Answer from the drawing. Dimensions are ordinates in mm from the lowest x, y and z of the part. A direction names the side the tool comes from. Round coordinates to 2 decimals unless told otherwise and drop trailing zeros. Order: outer loops, then holes, each group sorted by start corner. A loop starts at its lowest first (then second) coordinate and runs counter-clockwise, first axis right, second up.
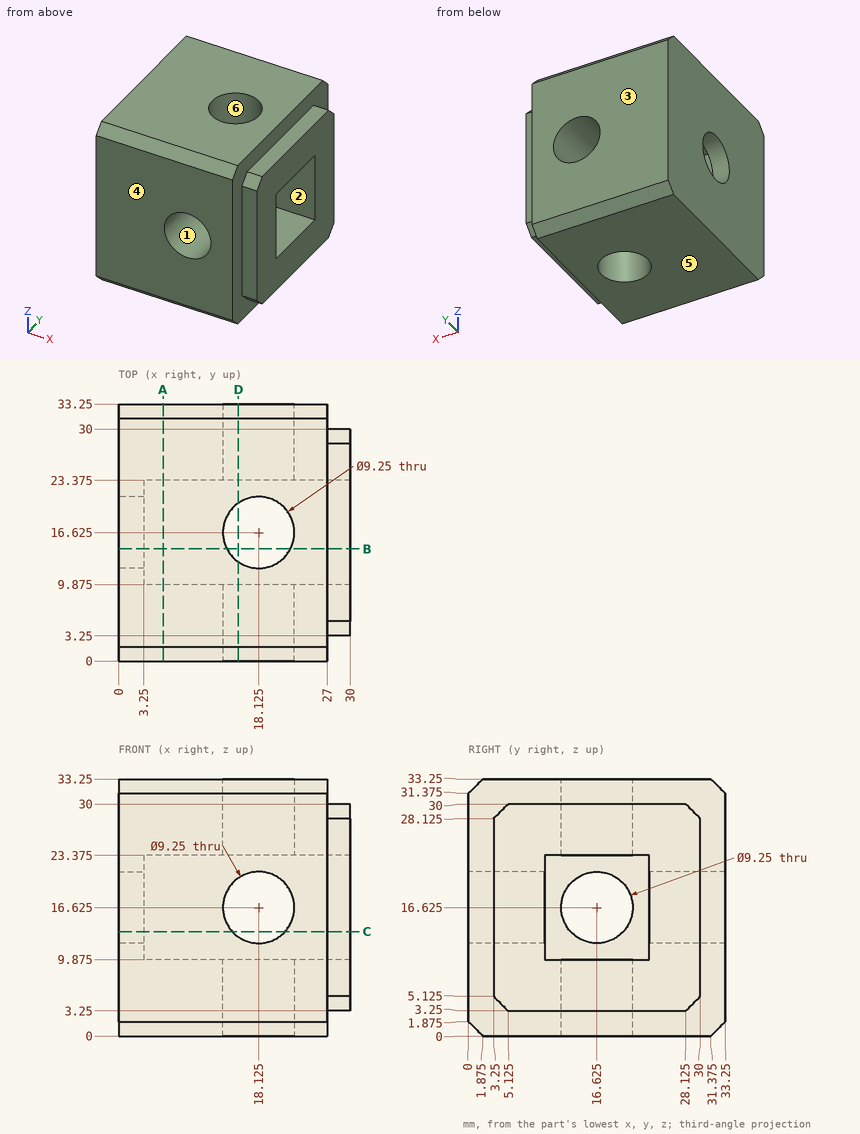
Q1. A cutting plane is placed at B-B, the plane y = 14.5. Give the vertices of the cut face in (x, z) (3 decimals).
Outcome:
outline: (0, 0) - (14.017, 0) - (14.017, 9.875) - (3.25, 9.875) - (3.25, 12.517) - (0, 12.517) - close; (0, 20.733) - (3.25, 20.733) - (3.25, 23.375) - (14.017, 23.375) - (14.017, 33.25) - (0, 33.25) - close; (22.233, 0) - (27, 0) - (27, 3.25) - (30, 3.25) - (30, 9.875) - (22.233, 9.875) - close; (22.233, 23.375) - (30, 23.375) - (30, 30) - (27, 30) - (27, 33.25) - (22.233, 33.25) - close
Q2. A cutting plane is placed at C-C, the plane z = 13.5. Give the vertices of the cut face in (x, y) (3 decimals), plus the area to 3 significant figures.
Outcome:
outline: (0, 0) - (14.715, 0) - (14.715, 9.875) - (3.25, 9.875) - (3.25, 13.215) - (0, 13.215) - close; (0, 20.035) - (3.25, 20.035) - (3.25, 23.375) - (14.715, 23.375) - (14.715, 33.25) - (0, 33.25) - close; (21.535, 0) - (27, 0) - (27, 3.25) - (30, 3.25) - (30, 9.875) - (21.535, 9.875) - close; (21.535, 23.375) - (30, 23.375) - (30, 30) - (27, 30) - (27, 33.25) - (21.535, 33.25) - close
area: 460 mm2
Q3. For the marked faces 1 and 2, determine the directions among +Z, -Z, +X, -X, +Y, -Y from which every point of the face is accessible in a straight line to the end or side of a thin tool.
Outcome:
face 1: +Y, -Y
face 2: +X
Q4. Straight lines are drawn through the part: probe 1 along X at (y, z) = (2, 16.5); probe 2 along Y at (x, z) = (6.5, 11.5) (3 decimals). For each, find the intervals that lie inside material, in ascending order.
Outcome:
probe 1: x = 0 to 13.5, 22.75 to 27
probe 2: y = 0 to 9.875, 23.375 to 33.25
Q5. For a pull along Y with two mould halves and no side action, classify the marked faces 3, 4, 5 and 6 as released by +Y, released by -Y, zero draft, split by the parting line, or undercut.
Outcome:
face 3: released by +Y
face 4: released by -Y
face 5: zero draft
face 6: undercut
Q6. Flat-ended cylindrical pins translate along their axes: pin 1 (0.9 mm diameter, centred on x = 28.5, z = 14, fed in from +Y); pin 2 (7.5 mm diameter, centred on x = 18.125, y = 16.625, fed in from -Z); pin 3 (2.5 mm diameter, centred on x = 28.5, y = 18, fed in from -Z). Find the tip coordinate at first contact, or state that the pin passes through.
Outcome:
pin 1: stops at y = 30
pin 2: passes through
pin 3: stops at z = 3.25
Q7. A cutting plane is placed at A-A, the plane x = 5.75. Give the vertices of the cut face in (y, z) (3 decimals).
Outcome:
outline: (0, 1.875) - (1.875, 0) - (31.375, 0) - (33.25, 1.875) - (33.25, 31.375) - (31.375, 33.25) - (1.875, 33.25) - (0, 31.375) - close; hole (9.875, 9.875) - (23.375, 9.875) - (23.375, 23.375) - (9.875, 23.375) - close
Q8. A cutting plane is placed at D-D, the plane x = 15.5. Give the vertices of the cut face in (y, z) (3 decimals), plus the area to 3 significant figures.
Outcome:
outline: (0, 1.875) - (1.875, 0) - (12.817, 0) - (12.817, 9.875) - (9.875, 9.875) - (9.875, 12.817) - (0, 12.817) - close; (0, 20.433) - (9.875, 20.433) - (9.875, 23.375) - (12.817, 23.375) - (12.817, 33.25) - (1.875, 33.25) - (0, 31.375) - close; (20.433, 0) - (31.375, 0) - (33.25, 1.875) - (33.25, 12.817) - (23.375, 12.817) - (23.375, 9.875) - (20.433, 9.875) - close; (20.433, 23.375) - (23.375, 23.375) - (23.375, 20.433) - (33.25, 20.433) - (33.25, 31.375) - (31.375, 33.25) - (20.433, 33.25) - close
area: 615 mm2
